```python
from build123d import *

# Parameters (mm, degrees)
SKETCH1_W           = 114
SKETCH1_H           = 67
BOSS_EXTRUDE1_DEPTH = 2.5
SKETCH2_W           = 2
SKETCH2_H           = 67
BOSS_EXTRUDE2_DEPTH = 18
LPATTERN1_COUNT     = 5
LPATTERN1_PITCH     = 19
SKETCH3_W           = 23
SKETCH3_H           = 67
BOSS_EXTRUDE3_DEPTH = 2


with BuildPart() as part:
    # Sketch1 → Boss-Extrude1 (new body, symmetric)
    with BuildSketch(Plane.XY):
        Rectangle(SKETCH1_W, SKETCH1_H)
    extrude(amount=BOSS_EXTRUDE1_DEPTH, both=True)

    # Sketch2 → Boss-Extrude2 (add)
    with BuildSketch(Plane.XY.offset(2.5)):
        with Locations((-38, 0)):
            Rectangle(SKETCH2_W, SKETCH2_H)
    boss_extrude2 = extrude(amount=BOSS_EXTRUDE2_DEPTH)

    # LPattern1: Boss-Extrude2 ×5
    with Locations(*[(i * LPATTERN1_PITCH, 0, 0) for i in range(1, LPATTERN1_COUNT)]):
        add(boss_extrude2)

    # Sketch3 → Boss-Extrude3 (add)
    with BuildSketch(Plane.ZY.offset(57)):
        with Locations((9, 0)):
            Rectangle(SKETCH3_W, SKETCH3_H)
    boss_extrude3 = extrude(amount=BOSS_EXTRUDE3_DEPTH)

    # Mirror1: Boss-Extrude3 across plane
    add(boss_extrude3.mirror(Plane(origin=(0, 0, 0), x_dir=(0, 0, 1), z_dir=(1, 0, 0))))


solid = part.part
```
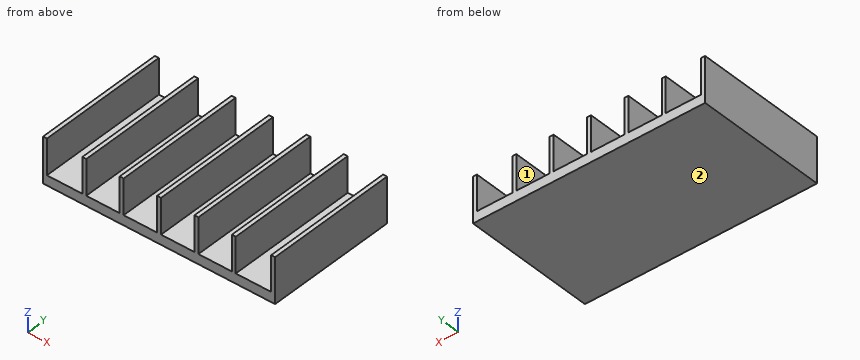
Work out the finished part from the listing and answer in its coordinate system (mm). Face numbers are marked on the shaded views. Give positions to 0.01 mm unless a question says otherwise; leave off trailing zeros. Order: outer loops, then holes, each group sorted by start corner. A loop starts at its lowest first (then second) coordinate and runs counter-clockwise, first axis right, second up. Notation, with made-up numbers: (0, 3.5) - (33, 3.5) arc R21 cw to (33, 38.5) - close; hole circle Ø6 at (-20.5, 5). An arc over 180 degrees is marked (long way). One line per item, written item: value. Start each with the question number.
1. Section A-A, the plane z = 10.25 is taken. Write down the section's boundary in (x, y).
2. Section C-C, the plane x = 11 is taken. Write down the section's boundary in (y, z).
3. Section B-B, the plane y = -29 is taken. Write down the section's boundary in (x, z), then the cut area to 3 significant figures.
4. This flat-tipped pin is pushed along its axis until it touches: pin 1 Ø5 at (x, y) = (13, -15) entering from +Z. Where does it stop, or does it pass through?
5. Consider line 1 (Z direction, x = 20.5, y = -3.5). Determine where the line is inside the solid, lowest interval first.
6. For a pull along X with two mould halves and no side action, classify the marked faces 1 and 2 as released by +X, released by -X, zero draft, split by the parting line, or undercut.
Filled sheet:
1. outline: (-59, -33.5) - (-57, -33.5) - (-57, 33.5) - (-59, 33.5) - close; (-39, -33.5) - (-37, -33.5) - (-37, 33.5) - (-39, 33.5) - close; (-20, -33.5) - (-18, -33.5) - (-18, 33.5) - (-20, 33.5) - close; (-1, -33.5) - (1, -33.5) - (1, 33.5) - (-1, 33.5) - close; (18, -33.5) - (20, -33.5) - (20, 33.5) - (18, 33.5) - close; (37, -33.5) - (39, -33.5) - (39, 33.5) - (37, 33.5) - close; (57, -33.5) - (59, -33.5) - (59, 33.5) - (57, 33.5) - close
2. outline: (-33.5, -2.5) - (33.5, -2.5) - (33.5, 2.5) - (-33.5, 2.5) - close
3. outline: (-59, -2.5) - (59, -2.5) - (59, 20.5) - (57, 20.5) - (57, 2.5) - (39, 2.5) - (39, 20.5) - (37, 20.5) - (37, 2.5) - (20, 2.5) - (20, 20.5) - (18, 20.5) - (18, 2.5) - (1, 2.5) - (1, 20.5) - (-1, 20.5) - (-1, 2.5) - (-18, 2.5) - (-18, 20.5) - (-20, 20.5) - (-20, 2.5) - (-37, 2.5) - (-37, 20.5) - (-39, 20.5) - (-39, 2.5) - (-57, 2.5) - (-57, 20.5) - (-59, 20.5) - close
3. area: 842 mm²
4. pin 1: z = 2.5
5. line 1: -2.5 to 2.5
6. face 1: undercut
6. face 2: zero draft
